For this review, take the finished solid that the model builds, in its own axes (mm). Round coordinates to 2 decimals unless told otherwise and drop trailing zeros. Write each loop counter-clockwise with the first axis right and the second up, starting at its lowest first coordinate (ties: lowest second). Pieces come first, ordered by that corner, then holes. Notation, with made-up numbers: (14, 87) - (33, 87) arc R26 ccw to (33, 111) - close; hole circle Ø2 at (50.5, 44.25). An arc over 180 degrees is marked (long way). One line per item, written item: value. Start each with the question number.
Q1. Clearance check with a flat-ended pin moving along its axis: pin 1 Ø1 at (y, z) = (-1.5, -13.5) entering from +X. State where the tip first meets the part, or that it passes through.
Q2. Add section A-A on z = -21. Write out the cut boundary in (x, y), and give its area (3 significant figures).
Q3. For probe 1 along X at (y, z) = (-0.1, 1); probe 2 along Y at (x, z) = (0.6, -15); probe 3 along Y at (x, z) = (1.65, -3), list the stretches that pass through material, from the lowest coordinate up.
```python
from build123d import *

# Parameters (mm, degrees)
SKETCH1_R           = 2
BOSS_EXTRUDE1_DEPTH = 27
FILLET1_R           = 1
FILLET2_R           = 1


with BuildPart() as part:
    # Sketch1 → Boss-Extrude1 (new body, symmetric)
    with BuildSketch(Plane.XY):
        Circle(SKETCH1_R)
    extrude(amount=BOSS_EXTRUDE1_DEPTH, both=True)

    # Fillet1
    fillet1_edges = [part.edges().sort_by_distance(p)[0] for p in [
        (-2, 0, 27),
    ]]
    fillet(fillet1_edges, radius=FILLET1_R)

    # Fillet2
    fillet2_edges = [part.edges().sort_by_distance(p)[0] for p in [
        (-2, 0, -27),
    ]]
    fillet(fillet2_edges, radius=FILLET2_R)


solid = part.part
```
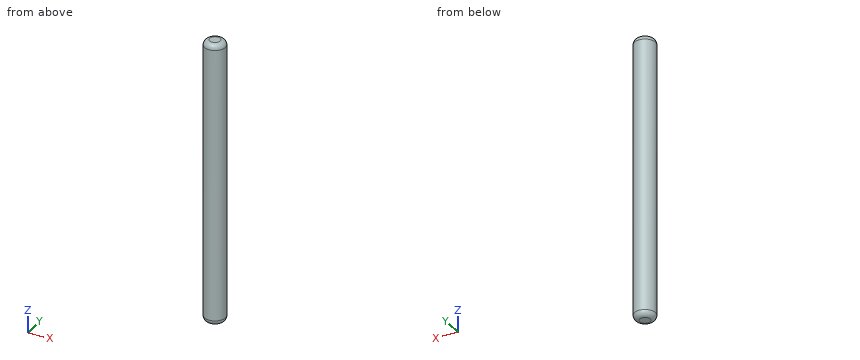
Result set:
1. pin 1: stops at x = 1.73
2. outline: circle Ø4 at (0, 0)
2. area: 12.6 mm^2
3. probe 1: x = -2 to 2
3. probe 2: y = -1.91 to 1.91
3. probe 3: y = -1.13 to 1.13
